from build123d import *

# Parameters (mm, degrees)
SKETCH1_R           = 9
BOSS_EXTRUDE3_DEPTH = 10
SKETCH54_R          = 12.040559159
BOSS_EXTRUDE5_DEPTH = 3.040559
BOSS_EXTRUDE5_TAPER = 45
SKETCH55_R          = 12.040559159
BOSS_EXTRUDE6_DEPTH = 3.040559
BOSS_EXTRUDE6_TAPER = 45
SKETCH56_R          = 12.040559159
BOSS_EXTRUDE7_DEPTH = 3.918882
SKETCH53_R          = 8
CUT_EXTRUDE7_DEPTH  = 11.0000001
SKETCH57_R          = 9
SKETCH57_R_2        = 8
CUT_EXTRUDE8_DEPTH  = 1
SKETCH59_R          = 9
SKETCH59_R_2        = 8
CUT_EXTRUDE9_DEPTH  = 1


with BuildPart() as part:
    # Sketch1 → Boss-Extrude3 (new body)
    with BuildSketch(Plane(origin=(0, 0, 0), x_dir=(1, 0, 0), z_dir=(0, 1, 0))):
        Circle(SKETCH1_R)
    extrude(amount=BOSS_EXTRUDE3_DEPTH)

    # Sketch54 → Boss-Extrude5 (add)
    with BuildSketch(Plane(origin=(0, 6.959440841, 0), x_dir=(1, 0, 0), z_dir=(0, 1, 0))):
        Circle(SKETCH54_R)
    extrude(amount=BOSS_EXTRUDE5_DEPTH, taper=BOSS_EXTRUDE5_TAPER)

    # Sketch55 → Boss-Extrude6 (add)
    with BuildSketch(Plane.XZ.offset(-3.040559159)):
        Circle(SKETCH55_R)
    extrude(amount=BOSS_EXTRUDE6_DEPTH, taper=BOSS_EXTRUDE6_TAPER)

    # Sketch56 → Boss-Extrude7 (add)
    with BuildSketch(Plane(origin=(0, 6.959440841, 0), x_dir=(-1, 0, 0), z_dir=(0, -1, 0))):
        Circle(SKETCH56_R)
    extrude(amount=BOSS_EXTRUDE7_DEPTH)

    # Sketch53 → Cut-Extrude7 (cut, through all)
    with BuildSketch(Plane(origin=(0, 10, 0), x_dir=(1, 0, 0), z_dir=(0, 1, 0))):
        Circle(SKETCH53_R)
    extrude(amount=-CUT_EXTRUDE7_DEPTH, mode=Mode.SUBTRACT)

    # Sketch57 → Cut-Extrude8 (cut)
    with BuildSketch(Plane(origin=(0, 0, 0), x_dir=(-1, 0, 0), z_dir=(0, -1, 0))):
        Circle(SKETCH57_R)
        Circle(SKETCH57_R_2, mode=Mode.SUBTRACT)
    extrude(amount=-CUT_EXTRUDE8_DEPTH, mode=Mode.SUBTRACT)

    # Sketch59 → Cut-Extrude9 (cut)
    with BuildSketch(Plane(origin=(0, 10, 0), x_dir=(1, 0, 0), z_dir=(0, 1, 0))):
        Circle(SKETCH59_R)
        Circle(SKETCH59_R_2, mode=Mode.SUBTRACT)
    extrude(amount=-CUT_EXTRUDE9_DEPTH, mode=Mode.SUBTRACT)


solid = part.part
Geometry check sheet. Reference: the model listing, model coordinates, mm. A direction names the side the tool comes from. Round coordinates to 2 decimals unless told otherwise and drop trailing zeros. Write each loop counter-clockwise with the first axis right and the second up, starting at its lowest first coordinate (ties: lowest second). Pieces come first, ordered by that corner, then holes. Notation, with made-up numbers: (86.25, 20.25) -> (93.25, 20.25) arc R11 cw to (93.25, 31.25) -> close; hole circle Ø11 at (36, 13.5). An arc over 180 degrees is marked (long way). One line per item, written item: value. Start each with the question number.
(1) Access from +Z, -Z, +X, -X, +Y, -Y to the whole of each face (thin tool, end or side, straight path). Record for faces 3 (the cylindrical face through (-1.172, 9.507, -8.923)), 4 (the cylindrical face through (-1.73, 5.06, 7.81)).
(2) Draft check along X on faces 1 (the cylindrical face through (1.172, 0.493, -8.923)), 2 (the cylindrical face through (2.61, 5.027, 11.754)). Enter one of: +X half, -X half, draft (parallel to the pull), parting line (faces both ways), or undercut.
(3) Go/stop test with flat-tipped pins: pin 1 Ø6 at (y, z) = (8, 8.5) entering from -X; pin 2 Ø1 at (x, y) = (8, 8) entering from -Z; pin 3 Ø9 at (x, z) = (4, -0.5) entering from +Y. Record where each tip stops, or that it passes through.
(4) Cross-section at B-B, the plane y = 5. Record the cut outline in (x, z), and give its area (3 significant figures).
(5) Cross-section at A-A, the plane x = 0. Record the cut outline in (y, z).
(6) Scan lines: line 1 (X direction, y = 3.5, z = 0); line 2 (Z direction, x = 0, y = 9.75); line 3 (X direction, y = 0.65, z = 0). Record each from-to range of solid material in increasing order. Write a range as [from, to].
Answer:
1. face 3: +Y
1. face 4: +Y, -Y
2. face 1: undercut
2. face 2: parting line
3. pin 1: x = -10.61
3. pin 2: z = -8.41
3. pin 3: y = 9
4. outline: circle Ø24.08 at (0, 0); hole circle Ø16 at (0, 0)
4. area: 254 mm²
5. outline: (0, -9) -> (3.04, -12.04) -> (6.96, -12.04) -> (10, -9) -> (9, -9) -> (9, -8) -> (1, -8) -> (1, -9) -> close; (0, 9) -> (1, 9) -> (1, 8) -> (9, 8) -> (9, 9) -> (10, 9) -> (6.96, 12.04) -> (3.04, 12.04) -> close
6. line 1: [-12.04, -8], [8, 12.04]
6. line 2: [-9.25, -9], [9, 9.25]
6. line 3: [-9.65, -9], [9, 9.65]
